from build123d import *

# Parameters (mm, degrees)
SKETCH1_W   = 40
SKETCH1_H   = 40
BLOCK_DEPTH = 44
SKETCH4_W   = 3.5
SKETCH4_H   = 0.8


# Read off the part's stored shape, not the designer's step: Hole
with BuildPart() as part:
    # Sketch1 → Block (new body)
    with BuildSketch(Plane(origin=(0, 0, 0), x_dir=(0, 1, 0), z_dir=(0, 0, 1))):
        Rectangle(SKETCH1_W, SKETCH1_H)
    extrude(amount=BLOCK_DEPTH)

    # Hole outline → Hole (revolve, cut)
    with BuildSketch(Plane.XZ):
        Polygon((0, 0), (3.8, 0), (3.4, 0.4), (3.4, 36), (0, 36), align=None)
    revolve(axis=Axis((0, 0, 0), (0, 0, 1)), mode=Mode.SUBTRACT)

    # Sketch4 → InsertGroove (revolve, cut)
    with BuildSketch(Plane(origin=(0, 0, 0), x_dir=(-1, 0, 0), z_dir=(0, 1, 0)), mode=Mode.PRIVATE) as insertgroove_sk:
        with Locations((-5.75, -0.1)):
            Rectangle(SKETCH4_W, SKETCH4_H)
    revolve(insertgroove_sk.sketch.rotate(Axis((0, 0, -200), (0, 0, 1)), 180), axis=Axis((0, 0, -200), (0, 0, 1)), mode=Mode.SUBTRACT)


solid = part.part
Part model, mm, in its own coordinate system. A direction names the side the tool comes from. Give positions to 0.01 mm unless a question says otherwise; leave off trailing zeros. Order: outer loops, then holes, each group sorted by start corner. A loop starts at its lowest first (then second) coordinate and runs counter-clockwise, first axis right, second up. Notation, with made-up numbers: (26, -24.5) - (41, -24.5) arc R30 ccw to (41, 9.5) - close; hole circle Ø5 at (80.5, 9.25). An arc over 180 degrees is marked (long way). One line per question, with ' | ' between items.
1. Pull direction X, two halves, no side cores. Call faces 1 (the face through (20, 0, 22)), 2 (the face through (-0.74, -3.32, 18.45)), 3 (the face through (0, -20, 22)): +X half, -X half, draft (parallel to the pull), parting line (faces both ways), or undercut.
Filled in:
face 1: +X half | face 2: undercut | face 3: draft
2. Which spindle directions (+Z, -Z, +X, -X, +Y, -Y) get a long thin tool onto all of the face, cutting with end or side? Do faces 4 (the face through (1.63, 7.32, 0.15)), 5 (the face through (0, 0, 44)). Say none if no direction does.
Filled in:
face 4: -Z | face 5: +Z, +X, -X, +Y, -Y
3. Band-saw the part on A-A on z = 23.5. List the corners of the cut face in (x, y), then the cut area to 3 significant figures.
Filled in:
outline: (-20, -20) - (20, -20) - (20, 20) - (-20, 20) - close; hole circle Ø6.8 at (0, 0) | area: 1,560 mm²
4. Drill centre lines: probe 1 along Y at (x, z) = (0, 19); probe 2 along X at (y, z) = (-3, 6); probe 3 along Z at (x, y) = (-0.5, -2.5). Where is each one in solid material? Low to high.
Filled in:
probe 1: -20 to -3.4, 3.4 to 20 | probe 2: -20 to -1.6, 1.6 to 20 | probe 3: 36 to 44
5. Band-saw the part on B-B on x = 0. List the corners of the cut face in (y, z).
Filled in:
outline: (-20, 0) - (-7.5, 0) - (-7.5, 0.3) - (-4, 0.3) - (-4, 0) - (-3.8, 0) - (-3.4, 0.4) - (-3.4, 36) - (3.4, 36) - (3.4, 0.4) - (3.8, 0) - (4, 0) - (4, 0.3) - (7.5, 0.3) - (7.5, 0) - (20, 0) - (20, 44) - (-20, 44) - close
